from build123d import *

# Parameters (mm, degrees)
F0_W         = 174
F0_H         = 110
F1_DEPTH     = 4
F2_W         = 174
F2_H         = 110
F2_W_2       = 168
F2_H_2       = 104
F3_DEPTH     = 46
F5_R         = 3.5
F6_DEPTH     = 2
F7_W         = 38.5
F7_H         = 15
F7_W_2       = 8
F7_H_2       = 17
F7_W_3       = 8.5
F7_H_3       = 6
F7_W_4       = 4
F7_H_4       = 5
F7_W_5       = 5
F7_H_5       = 12
F8_DEPTH     = 3
F9_W         = 9
F9_H         = 9
F9_R         = 1.63
F10_DEPTH    = 46
F11_DEPTH    = 50.001
F12_T1_DEPTH = 68.5
F13_R        = 3.63
F13_R_2      = 1.63
F14_DEPTH    = 2
F15_DEPTH    = 1.5


# Not quite as in the source:
# - a fillet or chamfer that OpenCascade refuses, or shapes differently, is made with other operations: its cross-section is extruded or revolved along the edge and cut away or added


with BuildPart() as f1:
    # F0 (on Top) → F1 (new body)
    with BuildSketch(Plane.XY):
        Rectangle(F0_W, F0_H)
    extrude(amount=-F1_DEPTH)

    # F2 (on face) → F3 (join)
    with BuildSketch(Plane.XY):
        Rectangle(F2_W, F2_H)
        Rectangle(F2_W_2, F2_H_2, mode=Mode.SUBTRACT)
    extrude(amount=F3_DEPTH)

    # F5 (on face) → F6 (cut)
    with BuildSketch(Plane(origin=(0, 0, -4), x_dir=(1, 0, 0), z_dir=(0, 0, -1))):
        with Locations((-66.7, 40.5)):
            Circle(F5_R)
        with Locations((-70, 26.5)):
            Circle(F5_R)
        with Locations((-66.7, -36.1)):
            Circle(F5_R)
        with Locations((-70, -46.5)):
            Circle(F5_R)
        with Locations((-5, -36.1)):
            Circle(F5_R)
        with Locations((5, -36.1)):
            Circle(F5_R)
        with Locations((-5, 40.5)):
            Circle(F5_R)
        with Locations((5, 40.5)):
            Circle(F5_R)
        with Locations((66.7, 40.5)):
            Circle(F5_R)
        with Locations((70, 26.5)):
            Circle(F5_R)
        with Locations((66.7, -36.1)):
            Circle(F5_R)
        with Locations((70, -46.5)):
            Circle(F5_R)
    extrude(amount=-F6_DEPTH, mode=Mode.SUBTRACT)

    # F7 (on face) → F8 (cut)
    with BuildSketch(Plane.XZ.offset(55)):
        with Locations((-52.75, 27.1)):
            Rectangle(F7_W, F7_H)
        with Locations((-14.25, 27.1)):
            Rectangle(F7_W, F7_H)
        with Locations((12, 28.1)):
            Rectangle(F7_W_2, F7_H_2)
        with Locations((20, 28.1)):
            Rectangle(F7_W_2, F7_H_2)
        with Locations((33.75, 22.6)):
            Rectangle(F7_W_3, F7_H_3)
        with Locations((42.25, 22.6)):
            Rectangle(F7_W_3, F7_H_3)
        with Locations((53, 22.1)):
            Rectangle(F7_W_4, F7_H_4)
        with Locations((57, 22.1)):
            Rectangle(F7_W_4, F7_H_4)
        with Locations((65.5, 25.6)):
            Rectangle(F7_W_5, F7_H_5)
        with Locations((70.5, 25.6)):
            Rectangle(F7_W_5, F7_H_5)
    extrude(amount=-F8_DEPTH, mode=Mode.SUBTRACT)

    # F9 (on face) → F10 (join)
    with BuildSketch(Plane.XY.offset(46)):
        with Locations((-79.5, 47.5)):
            Rectangle(F9_W, F9_H)
        with Locations((-81, 49)):
            Circle(F9_R, mode=Mode.SUBTRACT)
        Polygon((-75, 55), (-87, 55), (-87, 43), (-84, 43), (-84, 52), (-75, 52), align=None)
        Polygon((87, 55), (75, 55), (75, 52), (84, 52), (84, 43), (87, 43), align=None)
        with Locations((79.5, 47.5)):
            Rectangle(F9_W, F9_H)
        with Locations((81, 49)):
            Circle(F9_R, mode=Mode.SUBTRACT)
        Polygon((87, -55), (87, -43), (84, -43), (84, -52), (75, -52), (75, -55), align=None)
        with Locations((79.5, -47.5)):
            Rectangle(F9_W, F9_H)
        with Locations((81, -49)):
            Circle(F9_R, mode=Mode.SUBTRACT)
        with Locations((-79.5, -47.5)):
            Rectangle(F9_W, F9_H)
        with Locations((-81, -49)):
            Circle(F9_R, mode=Mode.SUBTRACT)
        Polygon((-84, -43), (-87, -43), (-87, -55), (-75, -55), (-75, -52), (-84, -52), align=None)
    extrude(amount=-F10_DEPTH)

    # F9 (on face) → F11 (cut, through all)
    with BuildSketch(Plane.XY.offset(46)):
        with Locations((-81, 49)):
            Circle(F9_R)
        with Locations((81, 49)):
            Circle(F9_R)
        with Locations((81, -49)):
            Circle(F9_R)
        with Locations((-81, -49)):
            Circle(F9_R)
    extrude(amount=-F11_DEPTH, mode=Mode.SUBTRACT)

    # F12: fillet of radius 10 on 4 edges, made by hand

    # F12_s2 → F12_t1 (cut)
    with BuildSketch(Plane.XY):
        with BuildLine():
            ThreePointArc((-75, 52), (-77.8832882455, 45.8832882455), (-84, 43))
            Line((-84, 43), (-75, 43))
            Line((-75, 43), (-75, 52))
        make_face()
        with BuildLine():
            ThreePointArc((84, 43), (77.8832882455, 45.8832882455), (75, 52))
            Line((75, 52), (75, 43))
            Line((75, 43), (84, 43))
        make_face()
        with BuildLine():
            ThreePointArc((-84, -43), (-77.8832882455, -45.8832882455), (-75, -52))
            Line((-75, -52), (-75, -43))
            Line((-75, -43), (-84, -43))
        make_face()
        with BuildLine():
            ThreePointArc((75, -52), (77.8832882455, -45.8832882455), (84, -43))
            Line((84, -43), (75, -43))
            Line((75, -43), (75, -52))
        make_face()
    extrude(amount=F12_T1_DEPTH, mode=Mode.SUBTRACT)

    # F13 (on face) → F14 (cut)
    with BuildSketch(Plane(origin=(0, 0, -4), x_dir=(1, 0, 0), z_dir=(0, 0, -1))):
        with Locations((-81, 49)):
            Circle(F13_R)
        with Locations((-81, 49)):
            Circle(F13_R_2, mode=Mode.SUBTRACT)
        with Locations((81, 49)):
            Circle(F13_R)
        with Locations((81, 49)):
            Circle(F13_R_2, mode=Mode.SUBTRACT)
        with Locations((81, -49)):
            Circle(F13_R)
        with Locations((81, -49)):
            Circle(F13_R_2, mode=Mode.SUBTRACT)
        with Locations((-81, -49)):
            Circle(F13_R)
        with Locations((-81, -49)):
            Circle(F13_R_2, mode=Mode.SUBTRACT)
    extrude(amount=-F14_DEPTH, mode=Mode.SUBTRACT)

    # F7 (on face) → F15 (cut)
    with BuildSketch(Plane.XZ.offset(55)):
        Polygon((-77, 34.6), (-77, 19.7916162387), (-77, 14.7916162387), (78, 14.7916162387), (78, 19.6), (78, 31.6), (78, 36.6), (73, 36.6), (68, 36.6), (63, 36.6), (59, 36.6), (59, 29.6), (55, 29.6), (51, 29.6), (46.5, 30.6), (38, 30.6), (29.5, 30.6), (29.5, 41.6), (24, 41.6), (16, 41.6), (8, 41.6), (5, 41.6), (5, 39.6), (-33.5, 39.6), (-72, 39.6), (-77, 39.6), align=None)
        Polygon((5, 19.6), (-33.5, 19.6), (-72, 19.6), (-72, 34.6), (-33.5, 34.6), (5, 34.6), align=None, mode=Mode.SUBTRACT)
        Polygon((46.5, 19.6), (38, 19.6), (29.5, 19.6), (29.5, 25.6), (38, 25.6), (46.5, 25.6), align=None, mode=Mode.SUBTRACT)
        Polygon((24, 19.6), (16, 19.6), (8, 19.6), (8, 36.6), (16, 36.6), (24, 36.6), align=None, mode=Mode.SUBTRACT)
        Polygon((59, 19.6), (55, 19.6), (51, 19.6), (51, 24.6), (55, 24.6), (59, 24.6), align=None, mode=Mode.SUBTRACT)
        Polygon((73, 19.6), (68, 19.6), (63, 19.6), (63, 31.6), (68, 31.6), (73, 31.6), align=None, mode=Mode.SUBTRACT)
    extrude(amount=-F15_DEPTH, mode=Mode.SUBTRACT)


solid = f1.part
Read the model definition and answer for the solid it produces. Units are mm, in the model's axes. A direction names the side the tool comes from. Coordinates: 2 decimals unless noted, no trailing zeros. Loops run counter-clockwise (first coordinate to the right, second up) from the corner with the lowest first, then second, coordinate; pieces in that order, holes last.
Q1. Consider probe 1 along Y at (x, z) = (81, -2.75); probe 2 along X at (y, z) = (36.1, -3.3); probe 3 along X at (y, z) = (49, -2.5). Determine where each line is inside the solid, lowest interval first.
Q2. The part is cut by section B-B on z = 7. Write down the section's boundary in (x, y), and give its area (3 significant figures).
Q3. The part is cut by section C-C on y = 15. Write down the section's boundary in (x, z), and give its area (3 significant figures).
Q4. Each of these flat-tipped pins is pushed along its axis until it touches: pin 1 Ø4 at (x, z) = (-8.5, 32) entering from -Y; pin 2 Ø1.5 at (x, y) = (-60, -14) entering from +Z; pin 3 Ø2 at (x, y) = (80.5, -49.5) entering from -Z. Where does it stop, or does it pass through?
Q5. The part is cut by section D-D on x = 61. Write down the section's boundary in (y, z), and give its area (3 significant figures).
Q6. The mould has two halves that part along X. Classify faces 4 (the face through (79.37, 49.07, 22.34)), 5 (the face through (87, -1, 21)), 6 (the face through (79.37, -48.93, 22.34)), 7 (the face through (-1, 55, 21)): +X half, -X half, draft (parallel to the pull), parting line (faces both ways), or undercut.
Q7. The part is cut by section A-A on x = -45. Write down the section's boundary in (y, z).
Q8. Which of the six approach directions +Z, -Z, +X, -X, +Y, -Y give full straight-line access (tool end or side, diameter ignored) to faces 1 (the face through (-82.63, -48.93, 22.34)), 2 (the face through (-1, 52, 23)), 3 (the face through (67.42, -28.865, -3.014))?
Results below:
1. probe 1: y = -55 to -52.63, -45.37 to 45.37, 52.63 to 55
1. probe 2: x = -87 to -70.2, -63.2 to -8.5, -1.5 to 1.5, 8.5 to 63.2, 70.2 to 87
1. probe 3: x = -87 to -84.63, -77.37 to -72.45, -67.55 to 67.55, 72.45 to 77.37, 84.63 to 87
2. outline: (-87, -55) - (87, -55) - (87, 55) - (-87, 55) - close; hole (-84, -43) arc R10 cw to (-75, -52) - (75, -52) arc R10 cw to (84, -43) - (84, 43) arc R10 cw to (75, 52) - (-75, 52) arc R10 cw to (-84, 43) - close; hole circle Ø3.26 at (-81, -49); hole circle Ø3.26 at (-81, 49); hole circle Ø3.26 at (81, -49); hole circle Ø3.26 at (81, 49)
2. area: 1,880 mm2
3. outline: (-87, -4) - (87, -4) - (87, 46) - (84, 46) - (84, 0) - (-84, 0) - (-84, 46) - (-87, 46) - close
3. area: 972 mm2
4. pin 1: stops at y = 52
4. pin 2: stops at z = 0
4. pin 3: stops at z = -2
5. outline: (-55, -4) - (55, -4) - (55, 46) - (52, 46) - (52, 0) - (-52, 0) - (-52, 46) - (-55, 46) - (-55, 36.6) - (-53.5, 36.6) - (-53.5, 14.79) - (-55, 14.79) - close
5. area: 683 mm2
6. face 4: undercut
6. face 5: +X half
6. face 6: undercut
6. face 7: draft
7. outline: (-55, -4) - (55, -4) - (55, 46) - (52, 46) - (52, 0) - (-52, 0) - (-52, 19.6) - (-53.5, 19.6) - (-53.5, 14.79) - (-55, 14.79) - close; (-55, 39.6) - (-53.5, 39.6) - (-53.5, 34.6) - (-52, 34.6) - (-52, 46) - (-55, 46) - close
8. face 1: +Z, -Z
8. face 2: +Z
8. face 3: -Z
